```python
from build123d import *

# Parameters (mm, degrees)
F0_R      = 0.254
F0_W      = 1.778
F0_H      = 3.81
F1_DEPTH  = 0.762
F3_R      = 0.254
F1_FACE_W = 5.334
F1_FACE_H = 0.762
F4_DEPTH  = 0.254


with BuildPart() as f1:
    # F0 (on Top) → F1 (new body)
    with BuildSketch(Plane.XY):
        Polygon((0.889, -2.667), (1.651, -2.667), (1.651, 2.667), (-1.651, 2.667), (-1.651, -2.667), (-0.889, -2.667), (-0.889, -28.067), (0.889, -28.067), align=None)
        with Locations((0, -27.305)):
            Circle(F0_R, mode=Mode.SUBTRACT)
        Rectangle(F0_W, F0_H, mode=Mode.SUBTRACT)
    extrude(amount=F1_DEPTH)

    # F3 (on offset) + F1_face (on face) → F4 (cut)
    with BuildSketch(Plane.YZ.offset(0.889)):
        with Locations((1.524, 0.381)):
            Circle(F3_R)
    with BuildSketch(Plane(origin=(1.651, 0, 0.381), x_dir=(0, 1, 0), z_dir=(1, 0, 0))):
        Rectangle(F1_FACE_W, F1_FACE_H)
    extrude(amount=F4_DEPTH, mode=Mode.SUBTRACT)


solid = f1.part
```
Check sheet for the modelled part. Datum: model origin and axes. Units: mm. Coordinates: 2 decimals unless noted, no trailing zeros. Write each loop counter-clockwise with the first axis right and the second up, starting at its lowest first coordinate (ties: lowest second). Pieces come first, ordered by that corner, then holes. Notation, with made-up numbers: M 10,26.5 L 61,26.5 A9 ccw 61,42.5 Z; hole C -10,29 d2. An arc over 180 degrees is marked long. Use one line per item in the form item = value.
Item 1: Sectioned sample at A-A, the plane x = 0. Record the cut outline in (y, z) (3 decimals), and give its area (3 significant figures).
Answer below:
outline = M -28.067,0 L -27.559,0 L -27.559,0.762 L -28.067,0.762 Z; M -27.051,0 L -1.905,0 L -1.905,0.762 L -27.051,0.762 Z; M 1.905,0 L 2.667,0 L 2.667,0.762 L 1.905,0.762 Z
area = 20.1 mm^2
Item 2: Sectioned sample at B-B, the plane x = 1.4. Record the cut outline in (y, z), and give its area (3 significant figures).
Answer below:
outline = M -2.67,0 L 2.67,0 L 2.67,0.76 L -2.67,0.76 Z
area = 4.06 mm^2
Item 3: Sectioned sample at C-C, the plane y = -4. Record the cut outline in (x, z).
Answer below:
outline = M -0.89,0 L 0.89,0 L 0.89,0.76 L -0.89,0.76 Z
Item 4: Material ranges on L1, parallel to Y at x = -0.05, z = 0.6 (3 decimals); L2, parallel to Y at x = 0.3, z = 0.2 (3 decimals); L3, parallel to X at y = 1.5, z = 0.6, recorded low to high. Write a range as from..to.
Answer below:
L1 = -28.067..-27.554, -27.056..-1.905, 1.905..2.667
L2 = -28.067..-1.905, 1.905..2.667
L3 = -1.65..-0.89, 1.14..1.65
